Build history of the part. All positions in model axes, mm. Face numbers are marked on the shaded views. A direction names the side the tool comes from. Give positions to 0.01 mm unless a question says otherwise; leave off trailing zeros. Order: outer loops, then holes, each group sorted by start corner. A loop starts at its lowest first (then second) coordinate and runs counter-clockwise, first axis right, second up. Notation, with made-up numbers: (26, 65.25) -> (30, 65.25) arc R23 cw to (30, 95.25) -> close; hole circle Ø9 at (-23.5, 6). An arc over 180 degrees is marked (long way). One line per question, with ' | ' between items. Start each with the question number.
(1) Drill centre lines: L1, parallel to Y at x = 0, z = 1.6; L2, parallel to Y at x = 0, z = 4.75; L3, parallel to Z at x = -15, y = -1.5. Where is each one in solid material? Low to high. Write a range as from..to.
(2) Pin check, flat tips, straight feed: pin 1 Ø1 at (y, z) = (-2, 6.5) entering from +X; pin 2 Ø6 at (x, z) = (-5.5, 4) entering from +Y; pin 3 Ø1.5 at (y, z) = (6.5, 3) entering from -X. Stop position of each tip, or through.
(3) Pull direction X, two halves, no side cores. Call the marked faces 1, 2 and 3: +X half, -X half, draft (parallel to the pull), parting line (faces both ways), or undercut.
(4) Cut at C-C (z = 9.25). Give the cut face in (x, y).
(5) Cut at D-D (x = 14.5). Give the cut face in (y, z), then the cut area to 3 significant figures.
(6) Which spindle directions (+Z, -Z, +X, -X, +Y, -Y) get a long thin tool onto all of the face, cutting with end or side? Do the marked faces 4 and 5. Say none if no direction does.
(7) Cut at B-B (x = 0). Give the cut face in (y, z), then the cut area to 3 significant figures.
(8) Cut at A-A (y = 0). Give the cut face in (x, z).
from build123d import *

# Parameters (mm, degrees)
SKETCH1_R               = 19
BOSS_EXTRUDE1_DEPTH     = 5
SKETCH2_R               = 3
BOSS_EXTRUDE2_DEPTH     = 7
SKETCH3_R               = 1.7
CUT_EXTRUDE1_DEPTH      = 30.427877939
SKETCH4_R               = 3
CUT_EXTRUDE2_DEPTH      = 2
CUT_EXTRUDE3_DEPTH      = 30.427877939
CUT_EXTRUDE3_DEPTH_BACK = 30.427877939
SKETCH5_R               = 1.7
SKETCH6_R               = 3
CUT_EXTRUDE4_DEPTH      = 2


with BuildPart() as part:
    # Sketch1 → Boss-Extrude1 (new body)
    with BuildSketch(Plane(origin=(0, 0, 0), x_dir=(0, 1, 0), z_dir=(0, 0, 1))):
        with Locations(Location((0, 0, 0), (0, 0, 270))):
            Circle(SKETCH1_R)
    extrude(amount=BOSS_EXTRUDE1_DEPTH)

    # Sketch2 → Boss-Extrude2 (add)
    with BuildSketch(Plane.XY.offset(5)):
        Circle(SKETCH2_R)
    extrude(amount=BOSS_EXTRUDE2_DEPTH)

    # Sketch3 → Cut-Extrude1 (cut, through all)
    with BuildSketch(Plane.XY.offset(12)):
        Circle(SKETCH3_R)
    extrude(amount=-CUT_EXTRUDE1_DEPTH, mode=Mode.SUBTRACT)

    # Sketch4 → Cut-Extrude2 (cut)
    with BuildSketch(Plane(origin=(0, 0, 0), x_dir=(1, 0, 0), z_dir=(0, 0, -1))):
        Circle(SKETCH4_R)
    extrude(amount=-CUT_EXTRUDE2_DEPTH, mode=Mode.SUBTRACT)

    # Sketch5 → Cut-Extrude3 (cut, two sides: drawn at the far end of the back side and taken through both)
    with BuildSketch(Plane(origin=(0, 0, 0), x_dir=(1, 0, 0), z_dir=(0, 0, -1)).offset(-CUT_EXTRUDE3_DEPTH_BACK)):
        with Locations((14, 0)):
            Circle(SKETCH5_R)
    extrude(amount=CUT_EXTRUDE3_DEPTH + CUT_EXTRUDE3_DEPTH_BACK, mode=Mode.SUBTRACT)

    # Sketch6 → Cut-Extrude4 (cut)
    with BuildSketch(Plane.XY.offset(5)):
        with Locations((14, 0)):
            Circle(SKETCH6_R)
    extrude(amount=-CUT_EXTRUDE4_DEPTH, mode=Mode.SUBTRACT)


solid = part.part
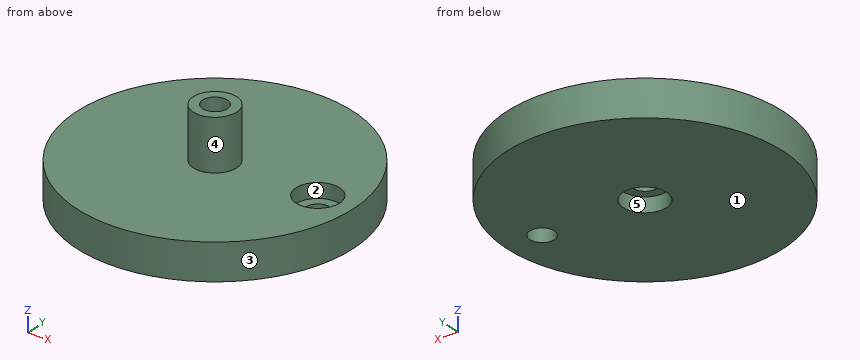
Result set:
1) L1: y = -19..-3, 3..19 | L2: y = -19..-1.7, 1.7..19 | L3: z = 0..5
2) pin 1: stops at x = 2.6 | pin 2: stops at y = 18.83 | pin 3: stops at x = -18.11
3) face 1: draft | face 2: undercut | face 3: parting line
4) outline: circle Ø6 at (0, 0); hole circle Ø3.4 at (0, 0)
5) outline: (-12.28, 0) -> (-1.62, 0) -> (-1.62, 3) -> (-2.96, 3) -> (-2.96, 5) -> (-12.28, 5) -> close; (1.62, 0) -> (12.28, 0) -> (12.28, 5) -> (2.96, 5) -> (2.96, 3) -> (1.62, 3) -> close | area: 101 mm2
6) face 4: +Z | face 5: -Z
7) outline: (-19, 0) -> (-3, 0) -> (-3, 2) -> (-1.7, 2) -> (-1.7, 12) -> (-3, 12) -> (-3, 5) -> (-19, 5) -> close; (1.7, 2) -> (3, 2) -> (3, 0) -> (19, 0) -> (19, 5) -> (3, 5) -> (3, 12) -> (1.7, 12) -> close | area: 186 mm2
8) outline: (-19, 0) -> (-3, 0) -> (-3, 2) -> (-1.7, 2) -> (-1.7, 12) -> (-3, 12) -> (-3, 5) -> (-19, 5) -> close; (1.7, 2) -> (3, 2) -> (3, 0) -> (12.3, 0) -> (12.3, 3) -> (11, 3) -> (11, 5) -> (3, 5) -> (3, 12) -> (1.7, 12) -> close; (15.7, 0) -> (19, 0) -> (19, 5) -> (17, 5) -> (17, 3) -> (15.7, 3) -> close
